from build123d import *

# Parameters (mm, degrees)
SKETCH1_W                 = 71
SKETCH1_H                 = 250
BOSS_EXTRUDE1_DEPTH       = 5
SKETCH2_W                 = 65
SKETCH2_H                 = 45
BOSS_EXTRUDE3_DEPTH       = 2
LPATTERN1_COUNT           = 3
LPATTERN1_PITCH           = 50
SKETCH3_W                 = 69
SKETCH3_H                 = 48.754858224
BOSS_EXTRUDE8_DEPTH       = 25
LPATTERN5_COUNT           = 3
LPATTERN5_PITCH           = 50
LPATTERN6_COUNT           = 2
LPATTERN6_PITCH           = 70
LPATTERN6_COPY_1_SKETCH_W = 65
LPATTERN6_COPY_1_SKETCH_H = 45
LPATTERN6_COPY_1_DEPTH    = 2
LPATTERN6_COPY_2_SKETCH_W = 65
LPATTERN6_COPY_2_SKETCH_H = 45
LPATTERN6_COPY_2_DEPTH    = 2
LPATTERN6_COPY_3_SKETCH_W = 69
LPATTERN6_COPY_3_SKETCH_H = 48.754858224
LPATTERN6_COPY_3_DEPTH    = 25
LPATTERN6_COPY_4_SKETCH_W = 69
LPATTERN6_COPY_4_SKETCH_H = 48.754858224
LPATTERN6_COPY_4_DEPTH    = 25
SKETCH6_W                 = 141
SKETCH6_H                 = 100.266772644
CUT_EXTRUDE1_DEPTH        = 10


with BuildPart() as part:
    # Sketch1 → Boss-Extrude1 (new body)
    with BuildSketch(Plane(origin=(0, 0, 0), x_dir=(1, 0, 0), z_dir=(0, 1, 0))):
        Rectangle(SKETCH1_W, SKETCH1_H)
    boss_extrude1 = extrude(amount=BOSS_EXTRUDE1_DEPTH)

    # Sketch2 → Boss-Extrude3 (add)
    with BuildSketch(Plane(origin=(0, 5, 0), x_dir=(1, 0, 0), z_dir=(0, 1, 0))):
        with Locations((0, -100)):
            Rectangle(SKETCH2_W, SKETCH2_H)
    boss_extrude3 = extrude(amount=BOSS_EXTRUDE3_DEPTH)

    # LPattern1: Boss-Extrude3 ×3
    with Locations(*[(0, 0, -i * LPATTERN1_PITCH) for i in range(1, LPATTERN1_COUNT)]):
        add(boss_extrude3)

    # Sketch3 → Boss-Extrude8 (add)
    with BuildSketch(Plane(origin=(0, 7, 0), x_dir=(1, 0, 0), z_dir=(0, 1, 0))):
        with Locations((0, -99.635002086)):
            Rectangle(SKETCH3_W, SKETCH3_H)
    boss_extrude8 = extrude(amount=BOSS_EXTRUDE8_DEPTH)

    # LPattern5: Boss-Extrude8 ×3
    with Locations(*[(0, 0, -i * LPATTERN5_PITCH) for i in range(1, LPATTERN5_COUNT)]):
        add(boss_extrude8)

    # LPattern6: Boss-Extrude1, Boss-Extrude3, Boss-Extrude8 ×2
    with Locations(*[(i * LPATTERN6_PITCH, 0, 0) for i in range(1, LPATTERN6_COUNT)]):
        add(boss_extrude1)
        add(boss_extrude3)
        add(boss_extrude8)

    # LPattern6 copy 1 sketch → LPattern6 copy 1 (add)
    with BuildSketch(Plane(origin=(70, 5, -50), x_dir=(1, 0, 0), z_dir=(0, 1, 0))):
        with Locations((0, -100)):
            Rectangle(LPATTERN6_COPY_1_SKETCH_W, LPATTERN6_COPY_1_SKETCH_H)
    extrude(amount=LPATTERN6_COPY_1_DEPTH)

    # LPattern6 copy 2 sketch → LPattern6 copy 2 (add)
    with BuildSketch(Plane(origin=(70, 5, -100), x_dir=(1, 0, 0), z_dir=(0, 1, 0))):
        with Locations((0, -100)):
            Rectangle(LPATTERN6_COPY_2_SKETCH_W, LPATTERN6_COPY_2_SKETCH_H)
    extrude(amount=LPATTERN6_COPY_2_DEPTH)

    # LPattern6 copy 3 sketch → LPattern6 copy 3 (add)
    with BuildSketch(Plane(origin=(70, 7, -50), x_dir=(1, 0, 0), z_dir=(0, 1, 0))):
        with Locations((0, -99.635002086)):
            Rectangle(LPATTERN6_COPY_3_SKETCH_W, LPATTERN6_COPY_3_SKETCH_H)
    extrude(amount=LPATTERN6_COPY_3_DEPTH)

    # LPattern6 copy 4 sketch → LPattern6 copy 4 (add)
    with BuildSketch(Plane(origin=(70, 7, -100), x_dir=(1, 0, 0), z_dir=(0, 1, 0))):
        with Locations((0, -99.635002086)):
            Rectangle(LPATTERN6_COPY_4_SKETCH_W, LPATTERN6_COPY_4_SKETCH_H)
    extrude(amount=LPATTERN6_COPY_4_DEPTH)

    # Sketch6 → Cut-Extrude1 (cut)
    with BuildSketch(Plane(origin=(0, 5, 0), x_dir=(1, 0, 0), z_dir=(0, 1, 0))):
        with Locations((35, 74.866613678)):
            Rectangle(SKETCH6_W, SKETCH6_H)
    extrude(amount=-CUT_EXTRUDE1_DEPTH, mode=Mode.SUBTRACT)


solid = part.part
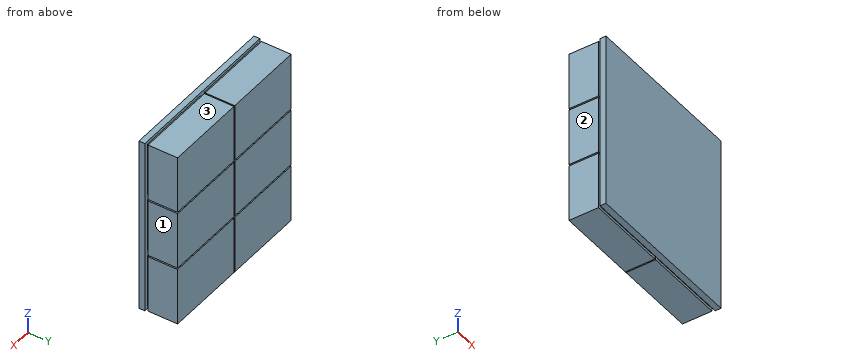
Source: CAD feature listing. Evaluate the final solid. Frame: model axes, mm. Face numbers are marked on the shaded views. A direction names the side the tool comes from. Give positions to 0.01 mm unless a question says otherwise; leave off trailing zeros. Loops run counter-clockwise (first coordinate to the right, second up) from the corner with the lowest first, then second, coordinate; pieces in that order, holes last. Notation, with made-up numbers: (24.5, -38.5) -> (35.5, -38.5) arc R20 ccw to (35.5, -28.5) -> close; hole circle Ø3 at (-20.75, 84). An arc over 180 degrees is marked (long way). Use a Markdown table: item, result. Add a question column.
1) Section query A-A, the plane z = 91.5. Return the cut outline in (x, y).
2) First-contact query: pin 1 (3 mm diameter, centred on x = 84, z = 51, fed in from -Y); pin 2 (0.6 mm diameter, centred on y = 5.5, z = 106, fed in from -X); pin 3 (1.6 mm diameter, centred on y = 6.5, z = 109, fed in from -X); pin 4 (0.6 mm diameter, centred on x = 0.5, y = 5.5, fed in from +Z). Flat tips, straight axial feed; report the tip coordinate or a pass-through.
3) Reachability of the marked faces 1, 2 and 3 from +Z, -Z, +X, -X, +Y, -Y: full face, straight path, thin tool, end or side. Return the list, or none.
4) Line query: line 1 along Z through (x, y) = (7, 29); line 2 along X through (y, z) = (31, 65); line 3 along Y through (x, z) = (3, 75.5). Output: solid intervals per line, ascending. Write a range as [from, to].
5) Section query C-C, the plane x = -22.5. Return the cut outline in (y, z), then the cut area to 3 significant figures.
6) Section query B-B, the plane y = 15.5. Return the cut outline in (x, z).
Numbers:
| question | item | result |
|---|---|---|
| 1 | outline | (-35.5, 0) -> (105.5, 0) -> (105.5, 5) -> (102.5, 5) -> (102.5, 7) -> (104.5, 7) -> (104.5, 32) -> (35.5, 32) -> (35.5, 7) -> (37.5, 7) -> (37.5, 5) -> (32.5, 5) -> (32.5, 7) -> (34.5, 7) -> (34.5, 32) -> (-34.5, 32) -> (-34.5, 7) -> (-32.5, 7) -> (-32.5, 5) -> (-35.5, 5) -> close |
| 2 | pin 1 | stops at y = 0 |
| 2 | pin 2 | stops at x = -32.5 |
| 2 | pin 3 | stops at x = -34.5 |
| 2 | pin 4 | stops at z = 122.5 |
| 3 | face 1 | +Z, -Z, +X, +Y |
| 3 | face 2 | +Z, -Z, -X, +Y |
| 3 | face 3 | +Z, +X, -X, +Y |
| 4 | line 1 | z = [-24.74, 24.01], [25.26, 74.01], [75.26, 124.01] |
| 4 | line 2 | x = [-34.5, 34.5], [35.5, 104.5] |
| 4 | line 3 | y = [0, 5], [7, 32] |
| 5 | outline | (0, -24.73) -> (5, -24.73) -> (5, -22.5) -> (7, -22.5) -> (7, -24.74) -> (32, -24.74) -> (32, 24.01) -> (7, 24.01) -> (7, 22.5) -> (5, 22.5) -> (5, 27.5) -> (7, 27.5) -> (7, 25.26) -> (32, 25.26) -> (32, 74.01) -> (7, 74.01) -> (7, 72.5) -> (5, 72.5) -> (5, 77.5) -> (7, 77.5) -> (7, 75.26) -> (32, 75.26) -> (32, 124.01) -> (7, 124.01) -> (7, 122.5) -> (5, 122.5) -> (5, 125) -> (0, 125) -> close |
| 5 | area | 4,680 mm2 |
| 6 | outline | (-34.5, -24.74) -> (34.5, -24.74) -> (34.5, 24.01) -> (-34.5, 24.01) -> close; (-34.5, 25.26) -> (34.5, 25.26) -> (34.5, 74.01) -> (-34.5, 74.01) -> close; (-34.5, 75.26) -> (34.5, 75.26) -> (34.5, 124.01) -> (-34.5, 124.01) -> close; (35.5, -24.74) -> (104.5, -24.74) -> (104.5, 24.01) -> (35.5, 24.01) -> close; (35.5, 25.26) -> (104.5, 25.26) -> (104.5, 74.01) -> (35.5, 74.01) -> close; (35.5, 75.26) -> (104.5, 75.26) -> (104.5, 124.01) -> (35.5, 124.01) -> close |
